Could you check a few things on this model? Use its own coordinates, in mm. A direction names the side the tool comes from. Round coordinates to 2 decimals unless told otherwise and drop trailing zeros. Write each loop counter-clockwise with the first axis right and the second up, starting at its lowest first coordinate (ties: lowest second). Pieces come first, ordered by that corner, then holes.
```python
from build123d import *

# Parameters (mm, degrees)
SKETCH1_W                = 40
SKETCH1_H                = 40
SKETCH1_H_2              = 10
SKETCH1_W_2              = 903
SKETCH1_H_3              = 2060
BOSS_EXTRUDE1_DEPTH      = 65
BOSS_EXTRUDE2_DEPTH      = 350
BOSS_EXTRUDE2_DEPTH_BACK = 50
SKETCH1_3_W              = 943
SKETCH1_3_H              = 80
SKETCH1_3_H_2            = 61
SKETCH1_4_W              = 40
SKETCH1_4_H              = 40
BOSS_EXTRUDE3_DEPTH      = 240
BOSS_EXTRUDE4_DEPTH      = 30
BOSS_EXTRUDE5_DEPTH      = 30
SKETCH5_W                = 30
SKETCH5_H                = 30
CUT_EXTRUDE1_DEPTH       = 200
BOSS_EXTRUDE6_DEPTH      = 30
BOSS_EXTRUDE7_START      = -30
BOSS_EXTRUDE7_DEPTH      = 30
BOSS_EXTRUDE8_DEPTH      = 15
BOSS_EXTRUDE8_DEPTH_BACK = 15
SKETCH8_W                = 683
SKETCH8_H                = 420
BOSS_EXTRUDE9_DEPTH      = 100


with BuildPart() as part:
    # Sketch1 → Boss-Extrude1 (new body)
    with BuildSketch(Plane(origin=(0, 0, 0), x_dir=(1, 0, 0), z_dir=(0, 1, 0))):
        with Locations((-431.5, 20)):
            Rectangle(SKETCH1_W, SKETCH1_H)
        Polygon((-411.5, 50), (-411.5, 40), (-411.5, 0), (411.5, 0), (411.5, 40), (411.5, 50), align=None)
        with Locations((-431.5, 45)):
            Rectangle(SKETCH1_W, SKETCH1_H_2)
        Polygon((-451.5, 0), (-451.5, 40), (-451.5, 50), (-451.5, 60), (-471.5, 60), (-471.5, -1), (471.5, -1), (471.5, 60), (451.5, 60), (451.5, 50), (451.5, 40), (451.5, 0), (411.5, 0), (-411.5, 0), align=None)
        Polygon((-451.5, 50), (-411.5, 50), (411.5, 50), (451.5, 50), (451.5, 60), (-451.5, 60), align=None)
        with Locations((431.5, 20)):
            Rectangle(SKETCH1_W, SKETCH1_H)
        with Locations((431.5, 45)):
            Rectangle(SKETCH1_W, SKETCH1_H_2)
        with Locations((0, 1090)):
            Rectangle(SKETCH1_W_2, SKETCH1_H_3)
        Polygon((-471.5, 2120), (-451.5, 2120), (-451.5, 2130), (-451.5, 2140), (-451.5, 2180), (-411.5, 2180), (411.5, 2180), (451.5, 2180), (451.5, 2140), (451.5, 2130), (451.5, 2120), (471.5, 2120), (471.5, 2200), (-471.5, 2200), align=None)
        Polygon((-451.5, 2130), (-451.5, 2120), (451.5, 2120), (451.5, 2130), (411.5, 2130), (-411.5, 2130), align=None)
        with Locations((-431.5, 2135)):
            Rectangle(SKETCH1_W, SKETCH1_H_2)
        with Locations((-431.5, 2160)):
            Rectangle(SKETCH1_W, SKETCH1_H)
        Polygon((-411.5, 2140), (-411.5, 2130), (411.5, 2130), (411.5, 2140), (411.5, 2180), (-411.5, 2180), align=None)
        with Locations((431.5, 2135)):
            Rectangle(SKETCH1_W, SKETCH1_H_2)
        with Locations((431.5, 2160)):
            Rectangle(SKETCH1_W, SKETCH1_H)
    extrude(amount=-BOSS_EXTRUDE1_DEPTH)

    # Sketch1_3 → Boss-Extrude2 (add, two sides: drawn at the far end of the back side and taken through both)
    with BuildSketch(Plane(origin=(0, 0, 0), x_dir=(1, 0, 0), z_dir=(0, 1, 0)).offset(-BOSS_EXTRUDE2_DEPTH_BACK)):
        with Locations((0, 2160)):
            Rectangle(SKETCH1_3_W, SKETCH1_3_H)
        with Locations((0, 29.5)):
            Rectangle(SKETCH1_3_W, SKETCH1_3_H_2)
    extrude(amount=BOSS_EXTRUDE2_DEPTH + BOSS_EXTRUDE2_DEPTH_BACK)

    # Sketch1_4 → Boss-Extrude3 (add)
    with BuildSketch(Plane(origin=(0, 0, 0), x_dir=(1, 0, 0), z_dir=(0, 1, 0))):
        with Locations((431.5, 2160)):
            Rectangle(SKETCH1_4_W, SKETCH1_4_H)
        with Locations((-431.5, 2160)):
            Rectangle(SKETCH1_4_W, SKETCH1_4_H)
        with Locations((-431.5, 20)):
            Rectangle(SKETCH1_4_W, SKETCH1_4_H)
        with Locations((431.5, 20)):
            Rectangle(SKETCH1_4_W, SKETCH1_4_H)
    extrude(amount=-BOSS_EXTRUDE3_DEPTH)

    # Sketch3 → Boss-Extrude4 (add)
    with BuildSketch(Plane(origin=(451.5, 0, 0), x_dir=(0, 0, -1), z_dir=(1, 0, 0))):
        Polygon((40, -65), (40, -205), (90, -205), (130, -65), align=None)
        Polygon((2140, -65), (2050, -65), (2090, -205), (2140, -205), align=None)
    extrude(amount=-BOSS_EXTRUDE4_DEPTH)

    # Sketch4 → Boss-Extrude5 (add)
    with BuildSketch(Plane(origin=(-451.5, 0, -45.75), x_dir=(0, 0, -1), z_dir=(1, 0, 0))):
        Polygon((2044.25, -205), (2094.25, -205), (2094.25, -65), (2004.25, -65), align=None)
        Polygon((44.25, -205), (84.25, -65), (-5.75, -65), (-5.75, -205), align=None)
    extrude(amount=BOSS_EXTRUDE5_DEPTH)

    # Sketch5 → Cut-Extrude1 (cut)
    with BuildSketch(Plane.XZ.offset(240)):
        with Locations((-431.5, -2160)):
            Rectangle(SKETCH5_W, SKETCH5_H)
        with Locations((431.5, -2160)):
            Rectangle(SKETCH5_W, SKETCH5_H)
        with Locations((431.5, -20)):
            Rectangle(SKETCH5_W, SKETCH5_H)
        with Locations((-431.5, -20)):
            Rectangle(SKETCH5_W, SKETCH5_H)
    extrude(amount=-CUT_EXTRUDE1_DEPTH, mode=Mode.SUBTRACT)

    # Sketch6 → Boss-Extrude6 (add)
    with BuildSketch(Plane.XY.offset(1)):
        with BuildLine():
            Line((130, -65), (-130, -65))
            ThreePointArc((-130, -65), (0, -195), (130, -65))
        make_face()
    extrude(amount=-BOSS_EXTRUDE6_DEPTH)

    # Sketch7 → Boss-Extrude7 (add)
    with BuildSketch(Plane(origin=(0, 0, -2200), x_dir=(-1, 0, 0), z_dir=(0, 0, -1)).offset(BOSS_EXTRUDE7_START)):
        with BuildLine():
            Line((130, -65), (-130, -65))
            ThreePointArc((-130, -65), (0, -195), (130, -65))
        make_face()
    extrude(amount=BOSS_EXTRUDE7_DEPTH)

    # 3DSketch1 → Boss-Extrude8 (add, two sides: drawn at the far end of the back side and taken through both)
    with BuildSketch(Plane(origin=(0, -195, -29), x_dir=(0, 0.014010768487145287, -0.9999018443659355), z_dir=(1, 0, 0)).offset(-BOSS_EXTRUDE8_DEPTH_BACK)):
        Polygon((0, 0), (0.420323055, 29.997055331), (2141.210171842, 0), (2140.789848787, -29.997055331), align=None)
    extrude(amount=BOSS_EXTRUDE8_DEPTH + BOSS_EXTRUDE8_DEPTH_BACK)

    # Sketch8 → Boss-Extrude9 (add)
    with BuildSketch(Plane.XZ.offset(65)):
        with Locations((0, -209)):
            Rectangle(SKETCH8_W, SKETCH8_H)
    extrude(amount=BOSS_EXTRUDE9_DEPTH)


solid = part.part
```
Q1. Imagine slicing it at B-B, the plane y = 131. Write out the boundary of the cut face in (x, z), then the cut area to 3 significant figures.
Q2. If I drill on L1, parallel to Z at x = 84.5, y = -107.5; L2, parallel to Z at x = 19, y = 254.5; L3, parallel to Y at x = -2, z = -1205.5, over which ranges is the centre line in solid material (lowest first)?
Q3. Imagine slicing it at D-D, the plane y = -144.5. Count the separate pieces of the cut face and the enclosed holes in it, then the cut area to 3 significant figures.
Q4. On a 3-axis mill with a long thin cutter (end or side, diameter ignored), from which of +Z, -Z, +X, -X, +Y, -Y can I reach the whole of each face in a straight line? I mean faces 1 (the flat face through (-421.5, -134, -74)), 2 (the flat face through (436.71, -135.98, -109.72)), 3 (the flat face through (411.5, -151, -2160)). Say none if no direction works.
Q5. Imagine slicing it at A-A, the plane z = -1543.5. Write out the boundary of the cut face in (x, y), then the cut area to 3 significant figures.
Q6. Imagine slicing it at C-C, the plane x = 297. Write out the boundary of the cut face in (y, z).
Q7. I'm going to push flat-ended pins straight in: pin 1 Ø15 at (x, z) = (-427.5, -2165.5) entering from -Y; pin 2 Ø20 at (y, z) = (-176, -24.5) entering from +X; pin 3 Ø4 at (x, z) = (-116.5, -574) entering from -Y. Where does each tip first touch, or does it pass through?
Q8. We'd pull the mould along X, two halves only. Please class faces 4 (the flat face through (471.5, 140, -2159)), 5 (the flat face through (431, -151, -2180)), 6 (the flat face through (421.5, -134, -74)): pulls with the +X half, pulls with the -X half, needs draft (parallel to the pull), parting line crosses it, or undercut.
Results found:
1. outline: (-471.5, -2200) - (471.5, -2200) - (471.5, -2120) - (-471.5, -2120) - close; (-471.5, -60) - (471.5, -60) - (471.5, 1) - (-471.5, 1) - close
1. area: 133,000 mm2
2. L1: z = -2200 to -2170, -419 to 1
2. L2: z = -2200 to -2120, -60 to 1
2. L3: y = -195 to -165, -65 to 0
3. separate pieces: 6
3. enclosed holes: 4
3. area: 304,000 mm2
4. face 1: -Y
4. face 2: +X, -Y
4. face 3: +Z, -Z, -Y
5. outline: (-451.5, -65) - (451.5, -65) - (451.5, 0) - (-451.5, 0) - close; (-15, -195) - (15, -195) - (15, -165) - (-15, -165) - close
5. area: 59,600 mm2
6. outline: (-165, -419) - (-65, -419) - (-65, -2200) - (350, -2200) - (350, -2120) - (0, -2120) - (0, -60) - (350, -60) - (350, 1) - (-165, 1) - close
7. pin 1: stops at y = -40
7. pin 2: stops at x = 451.5
7. pin 3: stops at y = -65
8. face 4: pulls with the +X half
8. face 5: needs draft
8. face 6: undercut
